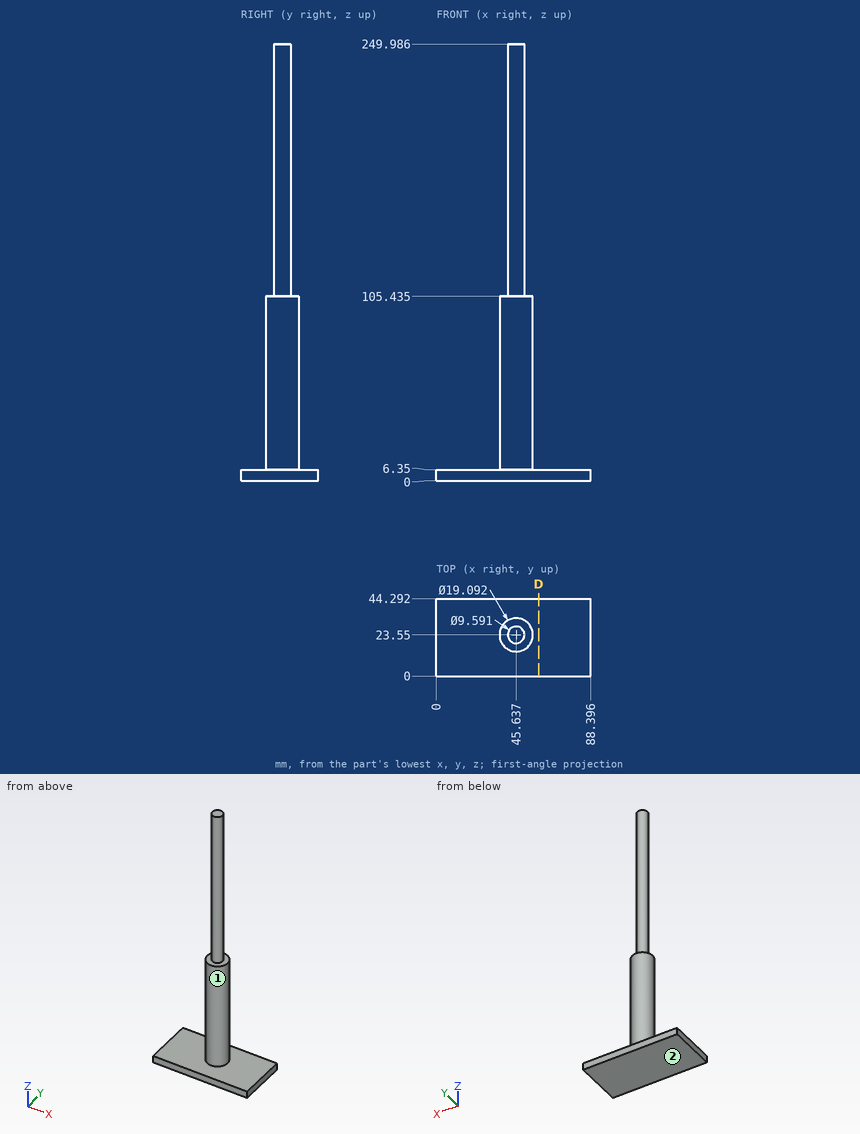
Here's the drawing with two shaded views (mm, measured from the low corner). I have some questions. A direction names the side the tool comes from. Give positions to 0.01 mm unless a question says otherwise; leave off trailing zeros. Loops run counter-clockwise (first coordinate to the right, second up) from the corner with the lowest first, then second, coordinate; pieces in that order, holes last. Notation, with made-up numbers: (56.5, 62) - (107.5, 62) arc R11 cw to (107.5, 72) - close; hole circle Ø1 at (-33.5, 73). An arc over 180 degrees is marked (long way). One line per item, written item: value.
(1) I'm going to push flat-ended pins straight in: pin 1 (12 mm diameter, centred on y = 24, z = 185, fed in from -X); pin 2 (5 mm diameter, centred on x = 25.5, y = 24.5, fed in from -Z); pin 3 (6 mm diameter, centred on x = 49, z = 210, fed in from +Y); pin 4 (3 mm diameter, centred on y = 24.5, z = 113, fed in from +X). Where does each tip first touch, or does it pass through?
Verdict:
pin 1: x = 40.84
pin 2: z = 0
pin 3: y = 28.33
pin 4: x = 50.43
(2) I need wall thicknesses on line 1 along Z through (x, y) = (70, 20.5); line 2 along X through (y, z) = (23, 192.5). Which ranges of each line are inside material? Lowest first, please.
Verdict:
line 1: 0 to 6.35
line 2: 40.87 to 50.4
(3) On a 3-axis mill with a long thin cutter (end or side, diameter ignored), from which of +Z, -Z, +X, -X, +Y, -Y can I reach the whole of each face in a straight line? I mean the marked faces 1 and 2. Say none if no direction works.
Verdict:
face 1: +Z
face 2: -Z, +X, -X, +Y, -Y
(4) If we section it at D-D, the plane x = 58.5: List the corners of the cut face in (y, z) for me, plus the area to 3 significant figures.
Verdict:
outline: (0, 0) - (44.29, 0) - (44.29, 6.35) - (0, 6.35) - close
area: 281 mm^2
